Geometry check sheet. Reference: drawing and pictorial views, mm from the part's lowest x, y, z. A direction names the side the tool comes from. Round coordinates to 2 decimals unless told otherwise and drop trailing zeros. Write each loop counter-clockwise with the first axis right and the second up, starting at its lowest first coordinate (ties: lowest second). Pieces come first, ordered by that corner, then holes. Notation, with made-up numbers: (1, 40) - (52, 40) arc R19 ccw to (52, 72) - close; hole circle Ø2 at (23, 2). An arc over 180 degrees is marked (long way). Return JSON: item names as keys, results as strings.
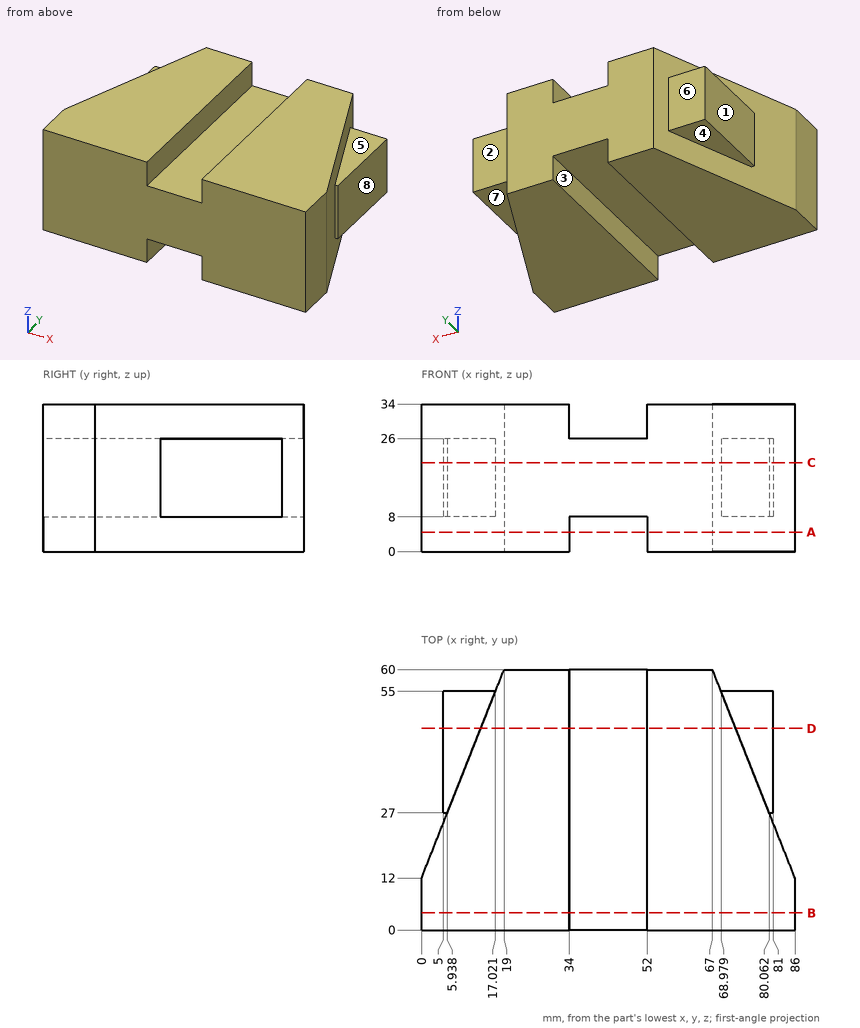
(1) Gauge pin test, flat ends, axial feed: pin 1 (6 mm diameter, centred on y = 52.5, z = 20, fed in from +X); pin 2 (3.5 mm diameter, centred on x = 8, z = 12.5, fed in from +Y); pin 3 (4 mm diameter, centred on y = 24.5, z = 5, fed in from -X). Record the tip position at first contact, or that the pin passes through.
Response values:
{"pin 1": "stops at x = 81", "pin 2": "stops at y = 55", "pin 3": "stops at x = 4.16"}
(2) Release check for a two-part mould opening along X. For the marked faces 1, 2 and 3 record: pulls with the +X half, pulls with the -X half, needs draft (parallel to the pull), parting line crosses it, or undercut.
Response values:
{"face 1": "pulls with the -X half", "face 2": "needs draft", "face 3": "undercut"}
(3) Section check A-A, the plane z = 4.5. Enter the section's corners in (x, y).
Response values:
{"outline": "(0, 0) - (34, 0) - (34, 60) - (19, 60) - (0, 12) - close; (52, 0) - (86, 0) - (86, 12) - (67, 60) - (52, 60) - close"}
(4) Access from +Z, -Z, +X, -X, +Y, -Y to the whole of each face (thin tool, end or side, straight path). Record for the marked faces 4, 5, 6, 7 and 8.
Response values:
{"face 4": "-Z, -X, +Y", "face 5": "+Z, +X, +Y", "face 6": "+Z, -Z, -X, +Y", "face 7": "-Z, +X, +Y", "face 8": "+Z, -Z, +X, +Y"}
(5) Material ranges on line 1 along X through (y, z) = (43.5, 22); line 2 along X through (y, z) = (12, 29.5); line 3 along Z through (x, y) = (79, 31), recorded low to high. Write a range as [from, to].
Response values:
{"line 1": "x = [5, 81]", "line 2": "x = [0, 34], [52, 86]", "line 3": "z = [8, 26]"}
(6) Section check C-C, the plane z = 20.5. Enter the section's corners in (x, y), plus the area to 3 significant figures.
Response values:
{"outline": "(0, 0) - (86, 0) - (86, 12) - (80.06, 27) - (81, 27) - (81, 55) - (68.98, 55) - (67, 60) - (19, 60) - (17.02, 55) - (5, 55) - (5, 27) - (5.94, 27) - (0, 12) - close", "area": "4,610 mm^2"}
(7) Section check D-D, the plane y = 46.5. Enter the section's corners in (x, z).
Response values:
{"outline": "(5, 8) - (13.66, 8) - (13.66, 0) - (34, 0) - (34, 8) - (52, 8) - (52, 0) - (72.34, 0) - (72.34, 8) - (81, 8) - (81, 26) - (72.34, 26) - (72.34, 34) - (52, 34) - (52, 26) - (34, 26) - (34, 34) - (13.66, 34) - (13.66, 26) - (5, 26) - close"}
(8) Section check B-B, the plane y = 4. Enter the section's corners in (x, z), plus the area to 3 significant figures.
Response values:
{"outline": "(0, 0) - (34, 0) - (34, 8) - (52, 8) - (52, 0) - (86, 0) - (86, 34) - (52, 34) - (52, 26) - (34, 26) - (34, 34) - (0, 34) - close", "area": "2,640 mm^2"}
